Autodesk Inventor part; units mm, degrees
ref_plane "Work Plane1" through (0, 5, 0) normal (0, 1, 0) x (1, 0, 0)
ref_plane "YZ Plane" through (0, 0, 0) normal (1, 0, 0) x (0, 1, 0)
ref_plane "XZ Plane" through (0, 0, 0) normal (0, 1, 0) x (-1, 0, 0)
sketch "Sketch1" plane through (0, 0, 0) normal (0, 1, 0) x (-1, 0, 0)
  line L0 (0, 0) -> (100, 0)
  line L1 (100, 0) -> (100, -70)
  line L2 (100, -70) -> (0, -70)
  line L3 (0, -70) -> (0, 0)
  dimension "d0" = 100
  dimension "d1" = 70
extrude "Extrusion1" add sketch "Sketch1" along normal blind 20
fillet "Fillet1" radius 15 2 edges at (-100, 20, -35) (0, 20, -35)
fillet "Fillet2" radius 5 10 edges at (-4.3934, 15.6066, 0) (0, 2.5, 0) (-95.6066, 15.6066, 0) (-100, 2.5, 0) (-50, 20, 0) (-95.6066, 15.6066, -70) (-100, 2.5, -70) (-4.3934, 15.6066, -70) (0, 2.5, -70) (-50, 20, -70)
shell "Shell1" thickness 2 removed faces 3 at (-0.0419, 6.121, -45) at (0, 1.6667, -25) at (-65, 0, -46.6667)
ref_plane "Work Plane1" through (0, 5, 0) normal (0, 1, 0) x (1, 0, 0)
sketch "Sketch2" plane through (0, 5, 0) normal (0, 1, 0) x (1, 0, 0)
  line L0 (-85, 65) -> (-15, 65) construction
  line L1 (-15, 65) -> (-15, 5) construction
  line L2 (-15, 5) -> (-85, 5) construction
  line L3 (-85, 5) -> (-85, 65) construction
  line L4 (-85, 5) -> (-85, 65) construction
  line L5 (-85, 35) -> (-15, 35) construction
  line L6 (-85, 35) -> (-75, 35) construction
  line L7 (-75, 35) -> (-75, 65) construction
  line L8 (-100, 65) -> (-100, 5) construction
  line L9 (-98, 65) -> (-98, 5) construction
  line L10 (-5, 70) -> (-95, 70) construction
  line L11 (-5, 68) -> (-95, 68) construction
  line L12 (-95, 2) -> (-5, 2) construction
  line L13 (-95, 0) -> (-5, 0) construction
  line L14 (-40, 35) -> (-40, 65) construction
  circle A0 centre (-75, 35) radius 3
  circle A1 centre (-40, 35) radius 3
  point P0 (0, 0)
  dimension "d9" = 25
  dimension "d10" = 35
  dimension "d11" = 6
  dimension "d12" = 6
extrude "Extrusion2" add sketch "Sketch2" along normal up to surface (13 mm away) draft 5
sketch "Sketch3" plane through (0, 20, 0) normal (0, 1, 0) x (1, 0, 0)
  circle A0 centre (-75, 35) radius 3 construction
  circle A1 centre (-75, 35) radius 4.1374 construction
  circle A2 centre (-40, 35) radius 3 construction
  circle A3 centre (-40, 35) radius 4.1374 construction
  line L0 (-85, 65) -> (-15, 65) construction
  line L1 (-85, 5) -> (-85, 65) construction
  line L2 (-15, 5) -> (-85, 5) construction
  line L3 (-15, 65) -> (-15, 5) construction
  point P0 (0, 0)
hole "Hole1" at (-75, 20, -35) direction (0, -1, 0) diameter 3.9 depth 15 countersink diameter 8.2 countersink angle 90
hole "Hole2" at (-40, 20, -35) direction (0, -1, 0) diameter 3.9 depth 15 countersink diameter 8.2 countersink angle 90
fillet "Fillet3" radius 1 2 edges at (-44.1374, 18, -35) (-79.1374, 18, -35)
sketch "Sketch4" plane through (0, 0, 0) normal (0, -1, 0) x (1, 0, 0)
  arc A0 (0, -5) -> (-5, 0) centre (-5, -5) ccw
  line L0 (-95, 0) -> (-5, 0)
  arc A1 (-95, 0) -> (-100, -5) centre (-95, -5) ccw
  line L1 (-100, -65) -> (-100, -5)
  arc A2 (-100, -65) -> (-95, -70) centre (-95, -65) ccw
  line L2 (-5, -70) -> (-95, -70)
  arc A3 (-5, -70) -> (0, -65) centre (-5, -65) ccw
  arc A4 (-1, -5) -> (-5, -1) centre (-5, -5) ccw
  line L3 (-5, -1) -> (-95, -1)
  arc A5 (-95, -1) -> (-99, -5) centre (-95, -5) ccw
  line L4 (-99, -5) -> (-99, -65)
  arc A6 (-99, -65) -> (-95, -69) centre (-95, -65) ccw
  line L5 (-95, -69) -> (-5, -69)
  arc A7 (-5, -69) -> (-1, -65) centre (-5, -65) ccw
  line L6 (-2, -5) -> (0, -5)
  line L7 (-1, -5) -> (0, -5)
  line L8 (0, -65) -> (-2, -65)
  line L9 (-1, -65) -> (0, -65)
  point P0 (0, 0)
  dimension "d30" = 1
extrude "Extrusion3" cut sketch "Sketch4" against normal blind 1
properties part number "A1.1"
Here's how the part is built. I have some questions about the finished solid (model axes, mm). A direction names the side the tool comes from. Coordinates: 2 decimals unless noted, no trailing zeros. Loops run counter-clockwise (first coordinate to the right, second up) from the corner with the lowest first, then second, coordinate; pieces in that order, holes last. Notation, with made-up numbers: (-34, 2) - (-2, 2) arc R15 cw to (-2, 13) - close; hole circle Ø11 at (63, 30). An arc over 180 degrees is marked (long way). Return JSON: item names as keys, results as strings. Group by question number.
Item 1: Will these pins go through, and if not, where does the flat tip stop? P1, Ø1, axis at x = -56.5, z = -50.5, coming from the -Y side; P2, Ø12, axis at y = 4.5, z = -41, coming from the +X side; P3, Ø6, axis at x = -75, z = -35, coming from the -Y side.
Item 2: We'd pull the mould along X, two halves only. Please class faces 1 (the face through (-2.203, 0.493, -67.859)), 2 (the face through (-95.72, 15.49, -35.42)), 3 (the face through (-38.27, 11.34, -34.1)): +X half, -X half, draft (parallel to the pull), parting line (faces both ways), or undercut.
Item 3: If we section it at A-A on z = -35: State how many separate pieces and enclosed holes the cut face has, and give its area (3 significant figures).
Item 4: If we section it at B-B on x = -40: Write out the boundary of the cut face in (y, z), and give its area (3 significant figures).
Item 5: If we section it at C-C on y = 2.5: Write out the boundary of the cut face in (x, z).
Item 6: On a 3-axis mill with a long thin cutter (end or side, diameter ignored), from which of +Z, -Z, +X, -X, +Y, -Y can I reach the whole of each face in a straight line? I mean faces 4 (the face through (-2.141, 0.493, -2.203)), 5 (the face through (-49.51, 17.1, -67.14)), 6 (the face through (-97.797, 0.493, -2.141)), 7 (the face through (-4, 13, -5)). Say none if no direction works.
Item 7: I need wall thicknesses on line 1 (Z direction, x = -32, y = 6.75); line 2 (Z direction, x = -40, y = 13.25); line 3 (X direction, y = 13, z = -35). Which ranges of each line are inside material? Lowest first, please. Write a range as from..to.
Item 8: If we section it at D-D on x = -52.5: Write out the boundary of the cut face in (y, z).
Calculated:
{
 "1": {"P1": "stops at y = 18", "P2": "stops at x = -36.87", "P3": "stops at y = 5"},
 "2": {"face 1": "+X half", "face 2": "-X half", "face 3": "undercut"},
 "3": {"separate pieces": "3", "enclosed holes": "0", "area": "253 mm^2"},
 "4": {"outline": "(0, -69) - (1, -69) - (1, -70) - (15, -70) arc R5 ccw to (20, -65) - (20, -39.1) - (17.85, -36.95) - (5, -36.95) - (5, -38) - (17.09, -39.06) arc R1 cw to (18, -40.05) - (18, -65) arc R3 cw to (15, -68) - (0, -68) - close; (0, -2) - (15, -2) arc R3 cw to (18, -5) - (18, -29.95) arc R1 cw to (17.09, -30.94) - (5, -32) - (5, -33.05) - (17.85, -33.05) - (20, -30.9) - (20, -5) arc R5 ccw to (15, 0) - (1, 0) - (1, -1) - (0, -1) - close", "area": "233 mm^2"},
 "5": {"outline": "(-100, -65) arc R5 ccw to (-95, -70) - (-5, -70) arc R5 ccw to (0, -65) - (-2, -65) arc R3 cw to (-5, -68) - (-95, -68) arc R3 cw to (-98, -65) - (-98, -5) arc R3 cw to (-95, -2) - (-5, -2) arc R3 cw to (-2, -5) - (0, -5) arc R5 ccw to (-5, 0) - (-95, 0) arc R5 ccw to (-100, -5) - close"},
 "6": {"face 4": "+Z, +X, -Y", "face 5": "-Y", "face 6": "+Z, -X, -Y", "face 7": "+X, +Y, -Y"},
 "7": {"line 1": "z = -70..-68, -2..0", "line 2": "z = -70..-68, -38.72..-36.95, -33.05..-31.28, -2..0", "line 3": "x = -97.69..-95.25, -78.7..-76.95, -73.05..-71.3, -43.7..-41.95, -38.05..-36.3"},
 "8": {"outline": "(0, -69) - (1, -69) - (1, -70) - (15, -70) arc R5 ccw to (20, -65) - (20, -5) arc R5 ccw to (15, 0) - (1, 0) - (1, -1) - (0, -1) - (0, -2) - (15, -2) arc R3 cw to (18, -5) - (18, -65) arc R3 cw to (15, -68) - (0, -68) - close"}
}
